Input: dimensioned drawing with shaded views. Units: mm. Origin: part minimum x, y, z. A direction names the side the tool comes from. Round coordinates to 2 decimals unless told otherwise and drop trailing zeros. Order: outer loops, then holes, each group sorted by start corner. A loop starts at its lowest first (then second) coordinate and runs counter-clockwise, first axis right, second up.
Item 1: Reachability of the marked faces 4, 5 and 6 from +Z, -Z, +X, -X, +Y, -Y: full face, straight path, thin tool, end or side. Return the list, or none.
Item 2: Cut plane B-B on z = 16.75. Output: boundary loops of the cut face in (x, y), then the cut area to 3 significant figures.
Item 3: Cut plane D-D on z = 2.5. Output: boundary loops of the cut face in (x, y), then the cut area to 3 significant figures.
Item 4: Mould query, pull axis X, two halves, no side actions, for the marked faces 1, 2 and 3. Classes: released by +X, released by -X, zero draft, split by the parting line, or undercut.
Item 5: Line query: L1, parallel to X at y = 0.5, z = 11; L2, parallel to X at y = 17, z = 18.25; L3, parallel to Z at x = 5, y = 1. Output: solid intervals per line, ascending.
Item 6: First-contact query: pin 1 (8 mm diameter, centred on y = 17.5, z = 20, fed in from -X); pin 2 (1 mm diameter, centred on y = 21.5, z = 7, fed in from +X). Flat tips, straight axial feed; report the tip coordinate or a pass-through.
Item 7: Cut plane A-A on x = 5. Output: boundary loops of the cut face in (y, z).
Item 8: Cut plane C-C on y = 14. Output: boundary loops of the cut face in (x, z), then the cut area to 3 significant figures.
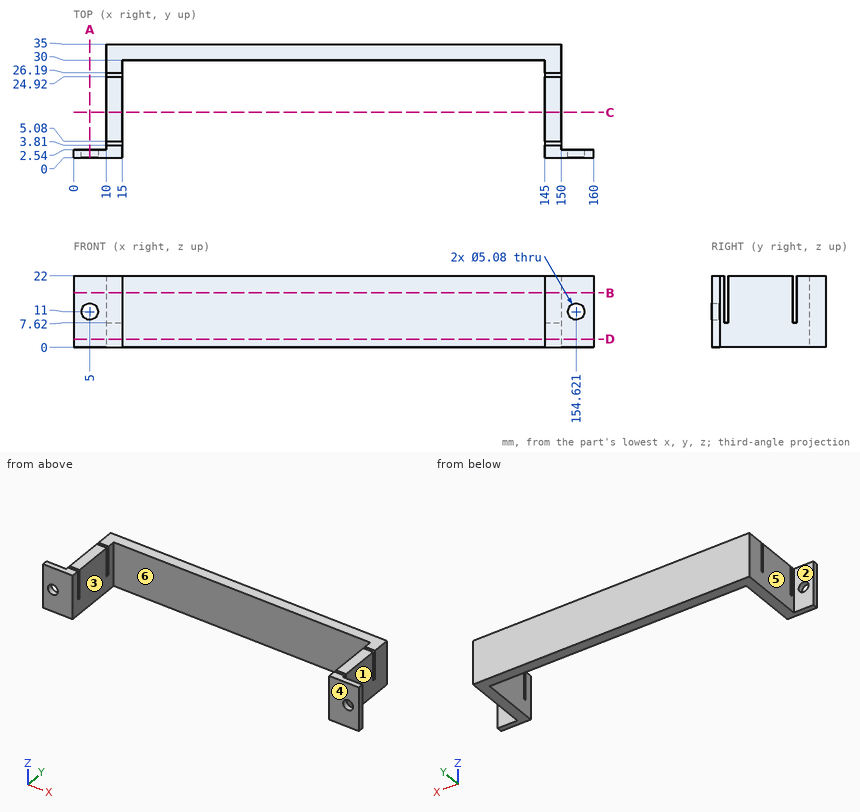
From the geometry:
1. face 4: +Z, -Z, +X, -X, -Y
1. face 5: +Z, -Z, -X, +Y
1. face 6: +Z, -Z, -Y
2. outline: (0, 0) - (15, 0) - (15, 3.81) - (10, 3.81) - (10, 2.54) - (0, 2.54) - close; (10, 5.08) - (15, 5.08) - (15, 24.92) - (10, 24.92) - close; (10, 26.19) - (15, 26.19) - (15, 30) - (145, 30) - (145, 26.19) - (150, 26.19) - (150, 35) - (10, 35) - close; (145, 0) - (160, 0) - (160, 2.54) - (150, 2.54) - (150, 3.81) - (145, 3.81) - close; (145, 5.08) - (150, 5.08) - (150, 24.92) - (145, 24.92) - close
2. area: 1,030 mm2
3. outline: (0, 0) - (15, 0) - (15, 30) - (145, 30) - (145, 0) - (160, 0) - (160, 2.54) - (150, 2.54) - (150, 35) - (10, 35) - (10, 2.54) - (0, 2.54) - close
3. area: 1,050 mm2
4. face 1: released by +X
4. face 2: zero draft
4. face 3: undercut
5. L1: x = 0 to 2.46, 7.54 to 15, 145 to 152.08, 157.16 to 160
5. L2: x = 10 to 15, 145 to 150
5. L3: z = 0 to 8.46, 13.54 to 22
6. pin 1: stops at x = 10
6. pin 2: stops at x = 150
7. outline: (0, 0) - (2.54, 0) - (2.54, 8.46) - (0, 8.46) - close; (0, 13.54) - (2.54, 13.54) - (2.54, 22) - (0, 22) - close
8. outline: (10, 0) - (15, 0) - (15, 22) - (10, 22) - close; (145, 0) - (150, 0) - (150, 22) - (145, 22) - close
8. area: 220 mm2
